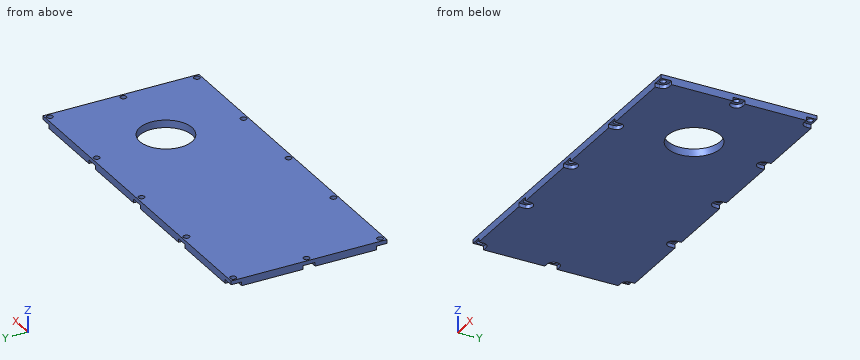
```python
from build123d import *

# Parameters (mm, degrees)
F0_R     = 23.5
F0_R_2   = 17.5
F1_DEPTH = 5
F0_R_3   = 2
F2_DEPTH = 2.5


# Not quite as in the source:
# - a feature names something its author has since deleted; it is built from what else it names


with BuildPart() as f1:
    # F0 (on Top) → F1 (new body)
    with BuildSketch(Plane.XY):
        with BuildLine():
            Line((-58.3766478719, 52), (-106.8995, 52))
            Line((-106.8995, 52), (-106.8995, 49))
            ThreePointArc((-106.8995, 49), (-108.1076845276, 46.0831845276), (-111.0245, 44.875))
            Line((-111.0245, 44.875), (-114.0245, 44.875))
            Line((-114.0245, 44.875), (-114.0245, 4.125))
            Line((-114.0245, 4.125), (-111.0245, 4.125))
            ThreePointArc((-111.0245, 4.125), (-106.8995, 0), (-111.0245, -4.125))
            Line((-111.0245, -4.125), (-114.0245, -4.125))
            Line((-114.0245, -4.125), (-114.0245, -44.875))
            Line((-114.0245, -44.875), (-111.0245, -44.875))
            ThreePointArc((-111.0245, -44.875), (-108.1076845276, -46.0831845276), (-106.8995, -49))
            Line((-106.8995, -49), (-106.8995, -52))
            Line((-106.8995, -52), (-58.3766478719, -52))
            Line((-58.3766478719, -52), (-58.3766478719, -47.5903098648))
            ThreePointArc((-58.3766478719, -47.5903098648), (-53.7843001577, -44.9375624638), (-50.375, -49))
            Line((-50.375, -49), (-50.375, -52))
            Line((-50.375, -52), (-4.125, -52))
            Line((-4.125, -52), (-4.125, -49))
            ThreePointArc((-4.125, -49), (0, -44.875), (4.125, -49))
            Line((4.125, -49), (4.125, -52))
            Line((4.125, -52), (50.375, -52))
            Line((50.375, -52), (50.375, -49))
            ThreePointArc((50.375, -49), (53.7843001577, -44.9375624638), (58.3766478719, -47.5903098648))
            Line((58.3766478719, -47.5903098648), (58.3766478719, -52))
            Line((58.3766478719, -52), (106.8995, -52))
            Line((106.8995, -52), (106.8995, -49))
            ThreePointArc((106.8995, -49), (108.1076845276, -46.0831845276), (111.0245, -44.875))
            Line((111.0245, -44.875), (114.0245, -44.875))
            Line((114.0245, -44.875), (114.0245, -4.125))
            Line((114.0245, -4.125), (111.0245, -4.125))
            ThreePointArc((111.0245, -4.125), (106.8995, 0), (111.0245, 4.125))
            Line((111.0245, 4.125), (114.0245, 4.125))
            Line((114.0245, 4.125), (114.0245, 44.875))
            Line((114.0245, 44.875), (111.0245, 44.875))
            ThreePointArc((111.0245, 44.875), (108.1076845276, 46.0831845276), (106.8995, 49))
            Line((106.8995, 49), (106.8995, 52))
            Line((106.8995, 52), (58.3766478719, 52))
            Line((58.3766478719, 52), (58.3766478719, 47.5903098648))
            ThreePointArc((58.3766478719, 47.5903098648), (53.7843001577, 44.9375624638), (50.375, 49))
            Line((50.375, 49), (50.375, 52))
            Line((50.375, 52), (4.125, 52))
            Line((4.125, 52), (4.125, 49))
            ThreePointArc((4.125, 49), (0, 44.875), (-4.125, 49))
            Line((-4.125, 49), (-4.125, 52))
            Line((-4.125, 52), (-50.375, 52))
            Line((-50.375, 52), (-50.375, 49))
            ThreePointArc((-50.375, 49), (-53.7843001577, 44.9375624638), (-58.3766478719, 47.5903098648))
            Line((-58.3766478719, 47.5903098648), (-58.3766478719, 52))
        make_face()
        with Locations((59.5245, 0)):
            Circle(F0_R, mode=Mode.SUBTRACT)
        with Locations((59.5245, 0)):
            Circle(F0_R)
        with Locations((59.5245, 0)):
            Circle(F0_R_2, mode=Mode.SUBTRACT)
    extrude(amount=-F1_DEPTH)

    # F0 (on Top) → F2 (join)
    with BuildSketch(Plane.XY):
        with BuildLine():
            Line((-106.8995, 52), (-114.0245, 52))
            Line((-114.0245, 52), (-114.0245, 44.875))
            Line((-114.0245, 44.875), (-111.0245, 44.875))
            ThreePointArc((-111.0245, 44.875), (-108.1076845276, 46.0831845276), (-106.8995, 49))
            Line((-106.8995, 49), (-106.8995, 52))
        make_face()
        with Locations((-111.0245, 49)):
            Circle(F0_R_3, mode=Mode.SUBTRACT)
        with BuildLine():
            Line((-111.0245, 4.125), (-114.0245, 4.125))
            Line((-114.0245, 4.125), (-114.0245, -4.125))
            Line((-114.0245, -4.125), (-111.0245, -4.125))
            ThreePointArc((-111.0245, -4.125), (-106.8995, 0), (-111.0245, 4.125))
        make_face()
        with Locations((-111.0245, 0)):
            Circle(F0_R_3, mode=Mode.SUBTRACT)
        with BuildLine():
            Line((-111.0245, -44.875), (-114.0245, -44.875))
            Line((-114.0245, -44.875), (-114.0245, -52))
            Line((-114.0245, -52), (-106.8995, -52))
            Line((-106.8995, -52), (-106.8995, -49))
            ThreePointArc((-106.8995, -49), (-108.1076845276, -46.0831845276), (-111.0245, -44.875))
        make_face()
        with Locations((-111.0245, -49)):
            Circle(F0_R_3, mode=Mode.SUBTRACT)
        with BuildLine():
            Line((-58.3766478719, -47.5903098648), (-58.3766478719, -52))
            Line((-58.3766478719, -52), (-50.375, -52))
            Line((-50.375, -52), (-50.375, -49))
            ThreePointArc((-50.375, -49), (-53.7843001577, -44.9375624638), (-58.3766478719, -47.5903098648))
        make_face()
        with Locations((-54.5, -49)):
            Circle(F0_R_3, mode=Mode.SUBTRACT)
        with BuildLine():
            Line((-4.125, -49), (-4.125, -52))
            Line((-4.125, -52), (4.125, -52))
            Line((4.125, -52), (4.125, -49))
            ThreePointArc((4.125, -49), (0, -44.875), (-4.125, -49))
        make_face()
        with Locations((0, -49)):
            Circle(F0_R_3, mode=Mode.SUBTRACT)
        with BuildLine():
            Line((50.375, -49), (50.375, -52))
            Line((50.375, -52), (58.3766478719, -52))
            Line((58.3766478719, -52), (58.3766478719, -47.5903098648))
            ThreePointArc((58.3766478719, -47.5903098648), (53.7843001577, -44.9375624638), (50.375, -49))
        make_face()
        with Locations((54.5, -49)):
            Circle(F0_R_3, mode=Mode.SUBTRACT)
        with BuildLine():
            Line((114.0245, -52), (114.0245, -44.875))
            Line((114.0245, -44.875), (111.0245, -44.875))
            ThreePointArc((111.0245, -44.875), (108.1076845276, -46.0831845276), (106.8995, -49))
            Line((106.8995, -49), (106.8995, -52))
            Line((106.8995, -52), (114.0245, -52))
        make_face()
        with Locations((111.0245, -49)):
            Circle(F0_R_3, mode=Mode.SUBTRACT)
        with BuildLine():
            Line((114.0245, -4.125), (114.0245, 4.125))
            Line((114.0245, 4.125), (111.0245, 4.125))
            ThreePointArc((111.0245, 4.125), (106.8995, 0), (111.0245, -4.125))
            Line((111.0245, -4.125), (114.0245, -4.125))
        make_face()
        with Locations((111.0245, 0)):
            Circle(F0_R_3, mode=Mode.SUBTRACT)
        with BuildLine():
            Line((114.0245, 52), (106.8995, 52))
            Line((106.8995, 52), (106.8995, 49))
            ThreePointArc((106.8995, 49), (108.1076845276, 46.0831845276), (111.0245, 44.875))
            Line((111.0245, 44.875), (114.0245, 44.875))
            Line((114.0245, 44.875), (114.0245, 52))
        make_face()
        with Locations((111.0245, 49)):
            Circle(F0_R_3, mode=Mode.SUBTRACT)
        with BuildLine():
            Line((58.3766478719, 52), (50.375, 52))
            Line((50.375, 52), (50.375, 49))
            ThreePointArc((50.375, 49), (53.7843001577, 44.9375624638), (58.3766478719, 47.5903098648))
            Line((58.3766478719, 47.5903098648), (58.3766478719, 52))
        make_face()
        with Locations((54.5, 49)):
            Circle(F0_R_3, mode=Mode.SUBTRACT)
        with BuildLine():
            Line((4.125, 52), (-4.125, 52))
            Line((-4.125, 52), (-4.125, 49))
            ThreePointArc((-4.125, 49), (0, 44.875), (4.125, 49))
            Line((4.125, 49), (4.125, 52))
        make_face()
        with Locations((0, 49)):
            Circle(F0_R_3, mode=Mode.SUBTRACT)
        with BuildLine():
            Line((-50.375, 52), (-58.3766478719, 52))
            Line((-58.3766478719, 52), (-58.3766478719, 47.5903098648))
            ThreePointArc((-58.3766478719, 47.5903098648), (-53.7843001577, 44.9375624638), (-50.375, 49))
            Line((-50.375, 49), (-50.375, 52))
        make_face()
        with Locations((-54.5, 49)):
            Circle(F0_R_3, mode=Mode.SUBTRACT)
    extrude(amount=-F2_DEPTH)


solid = f1.part
```
Model file for the job. Use its own axes, mm. Round coordinates to 2 decimals unless told otherwise and drop trailing zeros. Loops run counter-clockwise (first coordinate to the right, second up) from the corner with the lowest first, then second, coordinate; pieces in that order, holes last. Notation, with made-up numbers: M 16.25,-8 L 25.25,-8 A3 ccw 25.25,-3 Z; hole C 4,89 d3. An arc over 180 degrees is marked long. Put each result on its own line as item: value. Start each with the question number.
Item 1: Drop flat-ended pins along their axis: P1, Ø5, axis at x = 111.02, y = 0, coming from the -Z side; P2, Ø0.8, axis at y = 50.5, z = -3.5, coming from the +X side; P3, Ø0.8, axis at x = 112, z = -3.5, coming from the -Y side (3 decimals). Give the stop position or say it passes through.
Item 2: Drill centre lines: line 1 along Y through (x, z) = (-54.5, -1.2); line 2 along Y through (x, z) = (68, -1.1); line 3 along X through (y, z) = (-5.5, -3.7). Where is each one in solid material? Low to high.
Item 3: Cut at A-A (x = 68). List the corners of the cut face in (y, z), then the cut area to 3 significant figures.
Answer block:
1. P1: z = -2.5
1. P2: x = 106.9
1. P3: y = -44.875
2. line 1: -52 to -51, -47 to 47, 51 to 52
2. line 2: -52 to -15.31, 15.31 to 52
2. line 3: -114.02 to 42.91, 76.14 to 114.02
3. outline: M -52,-5 L -15.31,-5 L -15.31,0 L -52,0 Z; M 15.31,-5 L 52,-5 L 52,0 L 15.31,0 Z
3. area: 367 mm2
